Input: part model. Units: mm. Frame: model coordinates. A direction names the side the tool comes from. Give positions to 0.01 mm unless a question says otherwise; leave off trailing zeros. Loops run counter-clockwise (first coordinate to the right, second up) from the corner with the lowest first, then second, coordinate; pieces in that order, holes last. Notation, with made-up numbers: (7.5, -37.5) - (62.5, -37.5) arc R30 cw to (62.5, -13.5) - close; hole circle Ø2 at (-19.5, 17.5). An arc over 180 degrees is marked (long way). Answer as a JSON object with one key per item and string values.
from build123d import *

# Parameters (mm, degrees)
SKETCH1_W                = 28
SKETCH1_H                = 42
BOSS_EXTRUDE1_DEPTH      = 5
FILLET1_R                = 3
SKETCH3_R                = 1.585
CUT_EXTRUDE1_DEPTH       = 5
SKETCH4_W                = 14
SKETCH4_H                = 63
BOSS_EXTRUDE2_DEPTH      = 12
SKETCH5_W                = 14
SKETCH5_H                = 41
CUT_EXTRUDE2_DEPTH       = 3
SKETCH6_W                = 4
SKETCH6_H                = 8
BOSS_EXTRUDE3_DEPTH      = 18
SKETCH7_W                = 8
SKETCH7_H                = 27
BOSS_EXTRUDE4_DEPTH      = 10
SKETCH8_W                = 8
SKETCH8_H                = 27
BOSS_EXTRUDE5_DEPTH      = 10
BOSS_EXTRUDE6_DEPTH      = 10
BOSS_EXTRUDE6_DEPTH_BACK = 4
BOSS_EXTRUDE7_DEPTH      = 10
BOSS_EXTRUDE7_DEPTH_BACK = 4
CUT_EXTRUDE5_DEPTH       = 16
BOSS_EXTRUDE8_DEPTH      = 14
SKETCH16_R               = 2
CUT_EXTRUDE6_DEPTH       = 27
CUT_EXTRUDE8_START       = -8
SKETCH19_W               = 6
SKETCH19_H               = 14
CUT_EXTRUDE8_DEPTH       = 14
CUT_EXTRUDE9_DEPTH       = 1
CUT_EXTRUDE10_START      = -31
CUT_EXTRUDE10_DEPTH      = 3
CUT_EXTRUDE11_DEPTH      = 0.8
CUT_EXTRUDE12_START      = -13.2
CUT_EXTRUDE12_DEPTH      = 7.8
BOSS_EXTRUDE10_DEPTH     = 9


with BuildPart() as part:
    # Sketch1 → Boss-Extrude1 (new body)
    with BuildSketch(Plane(origin=(0, 0, 0), x_dir=(1, 0, 0), z_dir=(0, 1, 0))):
        Rectangle(SKETCH1_W, SKETCH1_H)
    extrude(amount=BOSS_EXTRUDE1_DEPTH)

    # Fillet1
    fillet1_edges = [part.edges().sort_by_distance(p)[0] for p in [
        (-14, 2.5, 21),
        (-14, 2.5, -21),
        (14, 2.5, -21),
        (14, 2.5, 21),
    ]]
    fillet(fillet1_edges, radius=FILLET1_R)

    # Sketch3 → Cut-Extrude1 (cut)
    with BuildSketch(Plane(origin=(0, 5, 0), x_dir=(1, 0, 0), z_dir=(0, 1, 0))):
        with Locations(Location((10, 18, 0), (0, 0, 270))):
            Circle(SKETCH3_R)
        with Locations(Location((-10, 18, 0), (0, 0, 270))):
            Circle(SKETCH3_R)
        with BuildLine():
            Line((1.585, -4.3), (1.585, -6.3))
            ThreePointArc((1.585, -6.3), (0, -7.885), (-1.585, -6.3))
            Line((-1.585, -6.3), (-1.585, -4.3))
            ThreePointArc((-1.585, -4.3), (0, -2.715), (1.585, -4.3))
        make_face()
    extrude(amount=-CUT_EXTRUDE1_DEPTH, mode=Mode.SUBTRACT)

    # Sketch4 → Boss-Extrude2 (add)
    with BuildSketch(Plane.XZ):
        with Locations((0, -30.5)):
            Rectangle(SKETCH4_W, SKETCH4_H)
    extrude(amount=BOSS_EXTRUDE2_DEPTH)

    # Sketch5 → Cut-Extrude2 (cut)
    with BuildSketch(Plane(origin=(0, 0, 0), x_dir=(1, 0, 0), z_dir=(0, 1, 0))):
        with Locations((0, 41.5)):
            Rectangle(SKETCH5_W, SKETCH5_H)
    extrude(amount=-CUT_EXTRUDE2_DEPTH, mode=Mode.SUBTRACT)

    # Sketch6 → Boss-Extrude3 (add)
    with BuildSketch(Plane.XZ.offset(12)):
        with Locations((-5, -58)):
            Rectangle(SKETCH6_W, SKETCH6_H)
        with Locations((5, -58)):
            Rectangle(SKETCH6_W, SKETCH6_H)
    extrude(amount=BOSS_EXTRUDE3_DEPTH)

    # Sketch7 → Boss-Extrude4 (add)
    with BuildSketch(Plane.ZY.offset(7)):
        with Locations((-58, -16.5)):
            Rectangle(SKETCH7_W, SKETCH7_H)
    extrude(amount=BOSS_EXTRUDE4_DEPTH)

    # Sketch8 → Boss-Extrude5 (add)
    with BuildSketch(Plane(origin=(7, 0, 0), x_dir=(0, 0, -1), z_dir=(1, 0, 0))):
        with Locations((58, -16.5)):
            Rectangle(SKETCH8_W, SKETCH8_H)
    extrude(amount=BOSS_EXTRUDE5_DEPTH)

    # Sketch9 → Boss-Extrude6 (add, two sides: drawn at the far end of the back side and taken through both)
    with BuildSketch(Plane.ZY.offset(7).offset(-BOSS_EXTRUDE6_DEPTH_BACK)):
        Polygon((-54, -30), (-42, -12), (-42, -3), (-54, -3), align=None)
    extrude(amount=BOSS_EXTRUDE6_DEPTH + BOSS_EXTRUDE6_DEPTH_BACK)

    # Sketch10 → Boss-Extrude7 (add, two sides: drawn at the far end of the back side and taken through both)
    with BuildSketch(Plane(origin=(7, 0, 0), x_dir=(0, 0, -1), z_dir=(1, 0, 0)).offset(-BOSS_EXTRUDE7_DEPTH_BACK)):
        Polygon((42, -12), (42, -3), (54, -3), (54, -30), align=None)
    extrude(amount=BOSS_EXTRUDE7_DEPTH + BOSS_EXTRUDE7_DEPTH_BACK)

    # Sketch13 → Cut-Extrude5 (cut)
    with BuildSketch(Plane.ZY.offset(7)):
        Polygon((1, 0), (-5, -12), (1, -12), align=None)
    extrude(amount=-CUT_EXTRUDE5_DEPTH, mode=Mode.SUBTRACT)

    # Sketch14 → Boss-Extrude8 (add)
    with BuildSketch(Plane.ZY.offset(7)):
        Polygon((-21, 0), (-22.5, -3), (-21, -3), align=None)
    extrude(amount=-BOSS_EXTRUDE8_DEPTH)

    # Sketch16 → Cut-Extrude6 (cut)
    with BuildSketch(Plane(origin=(0, 0, -62), x_dir=(-1, 0, 0), z_dir=(0, 0, -1))):
        with Locations((-10, -17)):
            Circle(SKETCH16_R)
        with Locations((-10, -25)):
            Circle(SKETCH16_R)
        with Locations((10, -17)):
            Circle(SKETCH16_R)
        with Locations((10, -25)):
            Circle(SKETCH16_R)
    extrude(amount=-CUT_EXTRUDE6_DEPTH, mode=Mode.SUBTRACT)

    # Sketch19 → Cut-Extrude8 (cut)
    with BuildSketch(Plane(origin=(0, 0, -62), x_dir=(-1, 0, 0), z_dir=(0, 0, -1)).offset(CUT_EXTRUDE8_START)):
        with Locations((-10, -21)):
            Rectangle(SKETCH19_W, SKETCH19_H)
        with Locations((10, -21)):
            Rectangle(SKETCH19_W, SKETCH19_H)
    extrude(amount=-CUT_EXTRUDE8_DEPTH, mode=Mode.SUBTRACT)

    # Sketch20 → Cut-Extrude9 (cut)
    with BuildSketch(Plane.ZY.offset(17)):
        Polygon((-60, -5), (-60, -27), (-54.40370085, -27), (-44, -11.394448725), (-44, -5), align=None)
        Polygon((-59, -6), (-59, -26), (-54.938884609, -26), (-45, -11.091673087), (-45, -6), align=None, mode=Mode.SUBTRACT)
    extrude(amount=-CUT_EXTRUDE9_DEPTH, mode=Mode.SUBTRACT)

    # Sketch24 → Cut-Extrude10 (cut)
    with BuildSketch(Plane.ZY.offset(17).offset(CUT_EXTRUDE10_START)):
        Polygon((-60, -5), (-60, -27), (-54.40370085, -27), (-44, -11.394448725), (-44, -5), align=None)
        Polygon((-59, -6), (-59, -26), (-54.938884609, -26), (-45, -11.091673087), (-45, -6), align=None, mode=Mode.SUBTRACT)
    extrude(amount=-CUT_EXTRUDE10_DEPTH, mode=Mode.SUBTRACT)

    # Sketch25 → Cut-Extrude11 (cut)
    with BuildSketch(Plane.ZY.offset(7)):
        Polygon((-40, -5), (-21.263932023, -5), (-19.763932023, -2), (-2.236067977, -2), (-6.236067977, -10), (-40, -10), align=None)
        Polygon((-39, -6), (-20.645898034, -6), (-19.145898034, -3), (-3.854101966, -3), (-6.854101966, -9), (-39, -9), align=None, mode=Mode.SUBTRACT)
    extrude(amount=-CUT_EXTRUDE11_DEPTH, mode=Mode.SUBTRACT)

    # Sketch26 → Cut-Extrude12 (cut)
    with BuildSketch(Plane.ZY.offset(7).offset(CUT_EXTRUDE12_START)):
        Polygon((-40, -5), (-21.263932023, -5), (-19.763932023, -2), (-2.236067977, -2), (-6.236067977, -10), (-40, -10), align=None)
        Polygon((-39, -6), (-20.645898034, -6), (-19.145898034, -3), (-3.854101966, -3), (-6.854101966, -9), (-39, -9), align=None, mode=Mode.SUBTRACT)
    extrude(amount=-CUT_EXTRUDE12_DEPTH, mode=Mode.SUBTRACT)

    # Sketch30 → Boss-Extrude10 (add)
    with BuildSketch(Plane.XZ.offset(12)):
        Polygon((-7, -42), (-7, -40.8), (-8.2, -42), align=None)
        Polygon((7, -42), (7, -40.8), (8.2, -42), align=None)
    extrude(amount=-BOSS_EXTRUDE10_DEPTH)


solid = part.part
Item 1: Material intervals for line 1 (X direction, y = 2.6, z = -18) (3 decimals); line 2 (Y direction, x = 6.5, z = -16.5); line 3 (X direction, y = -21, z = -49), sorted ascending. Write a range as [from, to].
Geometry check:
{"line 1": "x = [-14, -11.585], [-8.415, 8.415], [11.585, 14]", "line 2": "y = [-12, -10], [-9, -3], [-2, 5]", "line 3": "x = [-17, -13], [-7, -3], [3, 7], [13, 17]"}
Item 2: Contact query for flat-ended pins moving along their axis: P1, Ø8, axis at x = 6, z = -7, coming from the -Y side; P2, Ø1.5, axis at y = 1.5, z = 6, coming from the -X side; P3, Ø6, axis at y = -7, z = -27, coming from the -X side. Output: stop coordinate, or through.
Geometry check:
{"P1": "stops at y = -12", "P2": "stops at x = -14", "P3": "stops at x = -7"}
Item 3: Cut plane C-C (z = -1). Return loops of the section in (x, y), then the cut area to 3 significant figures.
Geometry check:
{"outline": "(-14, 0) - (-7, 0) - (-7, -4) - (7, -4) - (7, 0) - (14, 0) - (14, 5) - (-14, 5) - close", "area": "196 mm2"}
Item 4: Cut plane A-A (x = 10). Return loops of the section in (y, z) (3 decimals).
Geometry check:
{"outline": "(-30, -62) - (-27, -62) - (-27, -54) - (-28, -54) - (-28, -52.667) - (-30, -54) - close; (-23, -62) - (-19, -62) - (-19, -54) - (-23, -54) - close; (-15, -62) - (-3, -62) - (-3, -42) - (-12, -42) - (-14, -43.333) - (-14, -54) - (-15, -54) - close; (0, -21) - (5, -21) - (5, -19.585) - (0, -19.585) - close; (0, -16.415) - (5, -16.415) - (5, 21) - (0, 21) - close"}
Item 5: Cut plane B-B (x = -4). Return loops of the section in (y, z).
Geometry check:
{"outline": "(-30, -62) - (-3, -62) - (-3, -22.5) - (0, -21) - (5, -21) - (5, 21) - (0, 21) - (0, 1) - (-12, -5) - (-12, -42) - (-30, -54) - close"}
Item 6: Mould query, pull axis Y, two halves, no side actions, for faces 4 (the face through (14, 2, 0)), 5 (the face through (15.48, -18.65, -50.04)), 6 (the face through (0, -12, -27)). Classes: released by +Y, released by -Y, zero draft, split by the parting line, or undercut.
Geometry check:
{"face 4": "zero draft", "face 5": "undercut", "face 6": "released by -Y"}
Item 7: Cut plane D-D (y = -4). Return loops of the section in (x, z), then the cut area to 3 significant figures.
Geometry check:
{"outline": "(-17, -62) - (17, -62) - (17, -42) - (8.2, -42) - (7, -40.8) - (7, -20.76) - (6.2, -20.76) - (6.2, -19.65) - (7, -19.65) - (7, -4.35) - (6.2, -4.35) - (6.2, -3.24) - (7, -3.24) - (7, -1) - (-7, -1) - (-7, -3.24) - (-6.2, -3.24) - (-6.2, -4.35) - (-7, -4.35) - (-7, -19.65) - (-6.2, -19.65) - (-6.2, -20.76) - (-7, -20.76) - (-7, -40.8) - (-8.2, -42) - (-17, -42) - close", "area": "1,250 mm2"}
Item 8: Access query for faces 1 (the face through (-7, -4.6, -21.5)), 2 (the face through (13, -20, -50)), 3 (the face through (-1.585, 3, 5)). Directions: +Z, -Z, +X, -X, +Y, -Y. A direction counts if a zero-diameter tool reaches every point of the face in a straight line with its end or side. Return the directions, or none.
Geometry check:
{"face 1": "+Z, -X, -Y", "face 2": "+Z", "face 3": "+Y, -Y"}
